Geometry check sheet. Reference: the model listing, model coordinates, mm. Give positions to 0.01 mm unless a question says otherwise; leave off trailing zeros. Loops run counter-clockwise (first coordinate to the right, second up) from the corner with the lowest first, then second, coordinate; pieces in that order, holes last. Notation, with made-up numbers: (-20, -38.75) -> (11, -38.75) arc R32 cw to (11, -11.75) -> close; hole circle Ø9 at (45.25, 34). An arc over 180 degrees is marked (long way). Answer as a JSON object with one key per item and string values.
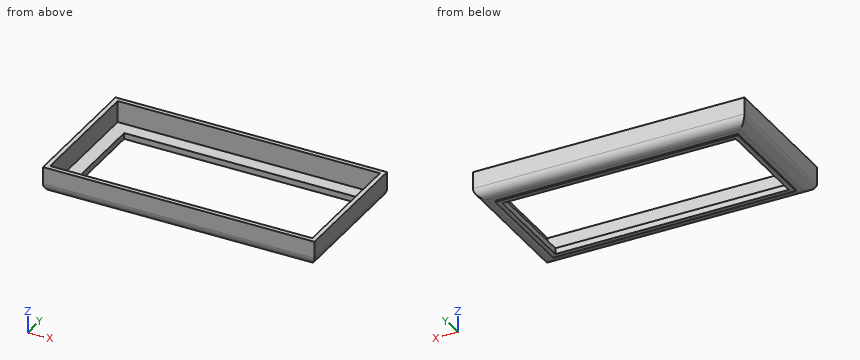
from build123d import *

# Parameters (mm, degrees)
F0_W     = 150.8212983608
F0_H     = 75.3069221973
F1_DEPTH = 14.5422648638
F2_W     = 134.8242838867
F2_H     = 60.1080209017
F3_DEPTH = 15.3549909592
F4_T     = -2.54
F5_R     = 5.08


with BuildPart() as f1:
    # F0 (on Top) → F1 (new body)
    with BuildSketch(Plane.XY):
        with Locations((75.4106491804, -37.6534610987)):
            Rectangle(F0_W, F0_H)
    extrude(amount=F1_DEPTH)

    # F2 (on face) → F3 (join)
    with BuildSketch(Plane.XY.offset(14.5422648638)):
        with Locations((75.1646866556, -37.8053411841)):
            Rectangle(F2_W, F2_H)
    extrude(amount=-F3_DEPTH)

    # F4
    f4_openings = [f1.faces().sort_by_distance(p)[0] for p in [
        (75.164687, -37.805341, -0.812726),
        (75.410649, -37.653461, 14.542265),
    ]]
    offset(amount=F4_T, openings=f4_openings, kind=Kind.INTERSECTION)

    # F5
    f5_edges = [f1.edges().sort_by_distance(p)[0] for p in [
        (75.410649, -75.306922, 0),
        (75.410649, 0, 0),
        (150.821298, -37.653461, 0),
        (0, -37.653461, 0),
    ]]
    fillet(f5_edges, radius=F5_R)


solid = f1.part
1) Section check B-B on x = 103. Record the cut outline in (y, z).
Geometry check:
{"outline": "(-75.31, 5.08) arc R5.08 ccw to (-70.23, 0) -> (-67.86, 0) -> (-67.86, -0.81) -> (-65.32, -0.81) -> (-65.32, 2.54) -> (-72.77, 2.54) -> (-72.77, 14.54) -> (-75.31, 14.54) -> close; (-10.29, -0.81) -> (-7.75, -0.81) -> (-7.75, 0) -> (-5.08, 0) arc R5.08 ccw to (0, 5.08) -> (0, 14.54) -> (-2.54, 14.54) -> (-2.54, 2.54) -> (-10.29, 2.54) -> close"}
2) Depth check by flat-ended pin: P1, Ø1.7, axis at y = -24, z = 0.5, coming from the +X side; P2, Ø0.7, axis at x = 50.5, z = -0.5, coming from the +Y side; P3, Ø6, axis at y = -46.5, z = 8.5, coming from the -X side; P4, Ø6, axis at x = 35.5, y = -61.5, coming from the -Z side. Enter the tip coordinate at first touch or a pass-through.
Geometry check:
{"P1": "stops at x = 149.19", "P2": "stops at y = -7.75", "P3": "stops at x = 0", "P4": "passes through"}
3) Section check C-C on z = 12.75. Record the cut outline in (x, y), plus the area to 3 significant figures.
Geometry check:
{"outline": "(0, -75.31) -> (150.82, -75.31) -> (150.82, 0) -> (0, 0) -> close; hole (2.54, -72.77) -> (148.28, -72.77) -> (148.28, -2.54) -> (2.54, -2.54) -> close", "area": "1,120 mm2"}
4) Material ranges on line 1 along Y through (x, z) = (43, 13.75); line 2 along X through (y, z) = (-36, 5); line 3 along X through (y, z) = (-58.5, 4.25), recorded low to high. Write a range as from..to.
Geometry check:
{"line 1": "y = -75.31..-72.77, -2.54..0", "line 2": "x = 0..2.54, 148.28..150.82", "line 3": "x = 0.07..2.54, 148.28..150.75"}
5) Section check A-A on y = -12. Record the cut outline in (x, z), plus the area to 3 significant figures.
Geometry check:
{"outline": "(0, 5.08) arc R5.08 ccw to (5.08, 0) -> (7.75, 0) -> (7.75, -0.81) -> (10.29, -0.81) -> (10.29, 2.54) -> (2.54, 2.54) -> (2.54, 14.54) -> (0, 14.54) -> close; (140.04, -0.81) -> (142.58, -0.81) -> (142.58, 0) -> (145.74, 0) arc R5.08 ccw to (150.82, 5.08) -> (150.82, 14.54) -> (148.28, 14.54) -> (148.28, 2.54) -> (140.04, 2.54) -> close", "area": "108 mm2"}
